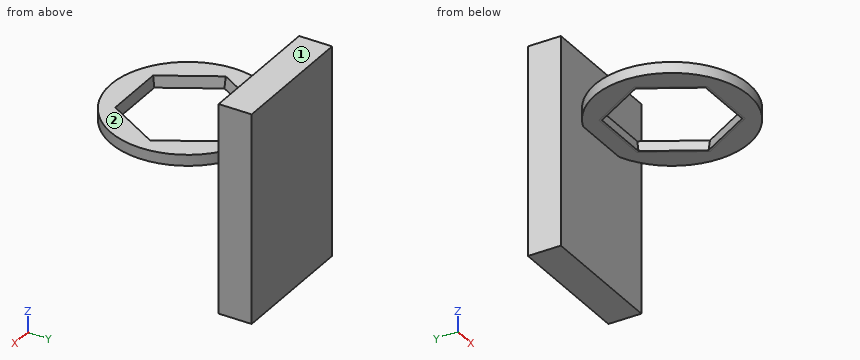
from build123d import *

# Parameters (mm, degrees)
ESQUISSE1_R               = 70
BOSS_EXTRU_1_DEPTH        = 10
CHANFREIN1_SIZE           = 10.000000024
CHANFREIN1_SIZE_2         = 1.74707794
D_PLACER_START            = -32.160153846
D_PLACER_LA_FACE1_DEPTH   = 61.565802755
D_PLACER_START_2          = -29.405648909
D_PLACER_LA_FACE1_2_DEPTH = 58.811297818
D_PLACER_LA_FACE1_3_DEPTH = 58.811297818
ESQUISSE2_W               = 120
ESQUISSE2_H               = 190
BOSS_EXTRU_2_DEPTH        = 30


with BuildPart() as part:
    # Esquisse1 → Boss.-Extru.1 (new body)
    with BuildSketch(Plane.XY):
        Circle(ESQUISSE1_R)
        Polygon((56.79394598, 0), (28.39697299, 49.185), (-28.39697299, 49.185), (-56.79394598, 0), (-28.39697299, -49.185), (28.39697299, -49.185), align=None, mode=Mode.SUBTRACT)
    extrude(amount=BOSS_EXTRU_1_DEPTH)

    # Chanfrein1
    # the kernel refuses this chamfer: 10.000000024, 1.74707794 mm, written as the material it takes off along each edge
    with BuildSketch(Plane(origin=(-54.38262227, -49.185, 10), x_dir=(0, 0, -1), z_dir=(1, 0, 0))) as chanfrein1_piece_1_section:
        Polygon((CHANFREIN1_SIZE, 0), (0, -CHANFREIN1_SIZE_2), (0, 0), align=None)
    chanfrein1_piece_1 = extrude(amount=108.76524454, mode=Mode.PRIVATE)
    chanfrein1_piece_1 = split(chanfrein1_piece_1, bisect_by=Plane(origin=(7.702074175, -85.029616205, 10), z_dir=(-0.8660254037844389, 0.4999999999999996, 0)), keep=Keep.TOP, mode=Mode.PRIVATE)
    chanfrein1_piece_1 = split(chanfrein1_piece_1, bisect_by=Plane(origin=(-34.89338531, -37.932883795, 10), z_dir=(0.8660254037844386, 0.5000000000000001, 0)), keep=Keep.TOP, mode=Mode.PRIVATE)
    add(chanfrein1_piece_1, mode=Mode.SUBTRACT)
    with BuildSketch(Plane(origin=(15.40414835, -71.68923241, 10), x_dir=(0, 0, -1), z_dir=(0.4999999999999996, 0.8660254037844389, 0))) as chanfrein1_piece_2_section:
        Polygon((CHANFREIN1_SIZE, 0), (0, -CHANFREIN1_SIZE_2), (0, 0), align=None)
    chanfrein1_piece_2 = extrude(amount=108.76524454, mode=Mode.PRIVATE)
    chanfrein1_piece_2 = split(chanfrein1_piece_2, bisect_by=Plane(origin=(15.40414835, -49.185, 10), z_dir=(0, 1, 0)), keep=Keep.TOP, mode=Mode.PRIVATE)
    chanfrein1_piece_2 = split(chanfrein1_piece_2, bisect_by=Plane(origin=(77.488844795, -35.844616205, 10), z_dir=(-0.8660254037844386, -0.5000000000000001, 0)), keep=Keep.TOP, mode=Mode.PRIVATE)
    add(chanfrein1_piece_2, mode=Mode.SUBTRACT)
    with BuildSketch(Plane(origin=(69.78677062, -22.50423241, 10), x_dir=(0, 0, -1), z_dir=(-0.5000000000000001, 0.8660254037844386, 0))) as chanfrein1_piece_3_section:
        Polygon((CHANFREIN1_SIZE, 0), (0, -CHANFREIN1_SIZE_2), (0, 0), align=None)
    chanfrein1_piece_3 = extrude(amount=108.76524454, mode=Mode.PRIVATE)
    chanfrein1_piece_3 = split(chanfrein1_piece_3, bisect_by=Plane(origin=(50.29753366, -11.252116205, 10), z_dir=(-0.8660254037844389, 0.4999999999999996, 0)), keep=Keep.TOP, mode=Mode.PRIVATE)
    chanfrein1_piece_3 = split(chanfrein1_piece_3, bisect_by=Plane(origin=(69.78677062, 49.185, 10), z_dir=(0, -1, 0)), keep=Keep.TOP, mode=Mode.PRIVATE)
    add(chanfrein1_piece_3, mode=Mode.SUBTRACT)
    with BuildSketch(Plane(origin=(54.38262227, 49.185, 10), x_dir=(0, 0, -1), z_dir=(-1, 0, 0))) as chanfrein1_piece_4_section:
        Polygon((CHANFREIN1_SIZE, 0), (0, -CHANFREIN1_SIZE_2), (0, 0), align=None)
    chanfrein1_piece_4 = extrude(amount=108.76524454, mode=Mode.PRIVATE)
    chanfrein1_piece_4 = split(chanfrein1_piece_4, bisect_by=Plane(origin=(-7.702074175, 85.029616205, 10), z_dir=(0.8660254037844388, -0.4999999999999998, 0)), keep=Keep.TOP, mode=Mode.PRIVATE)
    chanfrein1_piece_4 = split(chanfrein1_piece_4, bisect_by=Plane(origin=(34.89338531, 37.932883795, 10), z_dir=(-0.8660254037844386, -0.5000000000000001, 0)), keep=Keep.TOP, mode=Mode.PRIVATE)
    add(chanfrein1_piece_4, mode=Mode.SUBTRACT)
    with BuildSketch(Plane(origin=(-15.40414835, 71.68923241, 10), x_dir=(0, 0, -1), z_dir=(-0.4999999999999998, -0.8660254037844388, 0))) as chanfrein1_piece_5_section:
        Polygon((CHANFREIN1_SIZE, 0), (0, -CHANFREIN1_SIZE_2), (0, 0), align=None)
    chanfrein1_piece_5 = extrude(amount=108.76524454, mode=Mode.PRIVATE)
    chanfrein1_piece_5 = split(chanfrein1_piece_5, bisect_by=Plane(origin=(-77.488844795, 35.844616205, 10), z_dir=(0.8660254037844386, 0.5000000000000001, 0)), keep=Keep.TOP, mode=Mode.PRIVATE)
    chanfrein1_piece_5 = split(chanfrein1_piece_5, bisect_by=Plane(origin=(-15.40414835, 49.185, 10), z_dir=(0, -1, 0)), keep=Keep.TOP, mode=Mode.PRIVATE)
    add(chanfrein1_piece_5, mode=Mode.SUBTRACT)
    with BuildSketch(Plane(origin=(-69.78677062, 22.50423241, 10), x_dir=(0, 0, -1), z_dir=(0.5000000000000001, -0.8660254037844386, 0))) as chanfrein1_piece_6_section:
        Polygon((CHANFREIN1_SIZE, 0), (0, -CHANFREIN1_SIZE_2), (0, 0), align=None)
    chanfrein1_piece_6 = extrude(amount=108.76524454, mode=Mode.PRIVATE)
    chanfrein1_piece_6 = split(chanfrein1_piece_6, bisect_by=Plane(origin=(-69.78677062, -49.185, 10), z_dir=(0, 1, 0)), keep=Keep.TOP, mode=Mode.PRIVATE)
    chanfrein1_piece_6 = split(chanfrein1_piece_6, bisect_by=Plane(origin=(-50.29753366, 11.252116205, 10), z_dir=(0.8660254037844388, -0.4999999999999998, 0)), keep=Keep.TOP, mode=Mode.PRIVATE)
    add(chanfrein1_piece_6, mode=Mode.SUBTRACT)
    with BuildSketch(Plane(origin=(-54.38262227, -49.185, 10), x_dir=(0, 0, -1), z_dir=(1, 0, 0))) as chanfrein1_piece_7a_section:
        Polygon((CHANFREIN1_SIZE, 0), (0, -CHANFREIN1_SIZE_2), (0, 0), align=None)
    chanfrein1_piece_7a = extrude(amount=108.76524454, mode=Mode.PRIVATE)
    chanfrein1_piece_7a = split(chanfrein1_piece_7a, bisect_by=Plane(origin=(-34.89338531, -37.932883795, 10), z_dir=(-0.8660254037844386, -0.5000000000000001, 0)), keep=Keep.TOP, mode=Mode.PRIVATE)
    with BuildSketch(Plane(origin=(-69.78677062, 22.50423241, 10), x_dir=(0, 0, -1), z_dir=(0.5000000000000001, -0.8660254037844386, 0))) as chanfrein1_piece_7b_section:
        Polygon((CHANFREIN1_SIZE, 0), (0, -CHANFREIN1_SIZE_2), (0, 0), align=None)
    chanfrein1_piece_7b = extrude(amount=108.76524454, mode=Mode.PRIVATE)
    chanfrein1_piece_7b = split(chanfrein1_piece_7b, bisect_by=Plane(origin=(-69.78677062, -49.185, 10), z_dir=(0, -1, 0)), keep=Keep.TOP, mode=Mode.PRIVATE)
    chanfrein1_piece_7 = chanfrein1_piece_7a & chanfrein1_piece_7b
    add(chanfrein1_piece_7, mode=Mode.SUBTRACT)
    with BuildSketch(Plane(origin=(15.40414835, -71.68923241, 10), x_dir=(0, 0, -1), z_dir=(0.4999999999999996, 0.8660254037844389, 0))) as chanfrein1_piece_8a_section:
        Polygon((CHANFREIN1_SIZE, 0), (0, -CHANFREIN1_SIZE_2), (0, 0), align=None)
    chanfrein1_piece_8a = extrude(amount=108.76524454, mode=Mode.PRIVATE)
    chanfrein1_piece_8a = split(chanfrein1_piece_8a, bisect_by=Plane(origin=(15.40414835, -49.185, 10), z_dir=(0, -1, 0)), keep=Keep.TOP, mode=Mode.PRIVATE)
    with BuildSketch(Plane(origin=(-54.38262227, -49.185, 10), x_dir=(0, 0, -1), z_dir=(1, 0, 0))) as chanfrein1_piece_8b_section:
        Polygon((CHANFREIN1_SIZE, 0), (0, -CHANFREIN1_SIZE_2), (0, 0), align=None)
    chanfrein1_piece_8b = extrude(amount=108.76524454, mode=Mode.PRIVATE)
    chanfrein1_piece_8b = split(chanfrein1_piece_8b, bisect_by=Plane(origin=(7.702074175, -85.029616205, 10), z_dir=(0.8660254037844389, -0.4999999999999996, 0)), keep=Keep.TOP, mode=Mode.PRIVATE)
    chanfrein1_piece_8 = chanfrein1_piece_8a & chanfrein1_piece_8b
    add(chanfrein1_piece_8, mode=Mode.SUBTRACT)
    with BuildSketch(Plane(origin=(15.40414835, -71.68923241, 10), x_dir=(0, 0, -1), z_dir=(0.4999999999999996, 0.8660254037844389, 0))) as chanfrein1_piece_9a_section:
        Polygon((CHANFREIN1_SIZE, 0), (0, -CHANFREIN1_SIZE_2), (0, 0), align=None)
    chanfrein1_piece_9a = extrude(amount=108.76524454, mode=Mode.PRIVATE)
    chanfrein1_piece_9a = split(chanfrein1_piece_9a, bisect_by=Plane(origin=(77.488844795, -35.844616205, 10), z_dir=(0.8660254037844386, 0.5000000000000001, 0)), keep=Keep.TOP, mode=Mode.PRIVATE)
    with BuildSketch(Plane(origin=(69.78677062, -22.50423241, 10), x_dir=(0, 0, -1), z_dir=(-0.5000000000000001, 0.8660254037844386, 0))) as chanfrein1_piece_9b_section:
        Polygon((CHANFREIN1_SIZE, 0), (0, -CHANFREIN1_SIZE_2), (0, 0), align=None)
    chanfrein1_piece_9b = extrude(amount=108.76524454, mode=Mode.PRIVATE)
    chanfrein1_piece_9b = split(chanfrein1_piece_9b, bisect_by=Plane(origin=(50.29753366, -11.252116205, 10), z_dir=(0.8660254037844389, -0.4999999999999996, 0)), keep=Keep.TOP, mode=Mode.PRIVATE)
    chanfrein1_piece_9 = chanfrein1_piece_9a & chanfrein1_piece_9b
    add(chanfrein1_piece_9, mode=Mode.SUBTRACT)
    with BuildSketch(Plane(origin=(54.38262227, 49.185, 10), x_dir=(0, 0, -1), z_dir=(-1, 0, 0))) as chanfrein1_piece_10a_section:
        Polygon((CHANFREIN1_SIZE, 0), (0, -CHANFREIN1_SIZE_2), (0, 0), align=None)
    chanfrein1_piece_10a = extrude(amount=108.76524454, mode=Mode.PRIVATE)
    chanfrein1_piece_10a = split(chanfrein1_piece_10a, bisect_by=Plane(origin=(34.89338531, 37.932883795, 10), z_dir=(0.8660254037844386, 0.5000000000000001, 0)), keep=Keep.TOP, mode=Mode.PRIVATE)
    with BuildSketch(Plane(origin=(69.78677062, -22.50423241, 10), x_dir=(0, 0, -1), z_dir=(-0.5000000000000001, 0.8660254037844386, 0))) as chanfrein1_piece_10b_section:
        Polygon((CHANFREIN1_SIZE, 0), (0, -CHANFREIN1_SIZE_2), (0, 0), align=None)
    chanfrein1_piece_10b = extrude(amount=108.76524454, mode=Mode.PRIVATE)
    chanfrein1_piece_10b = split(chanfrein1_piece_10b, bisect_by=Plane(origin=(69.78677062, 49.185, 10), z_dir=(0, 1, 0)), keep=Keep.TOP, mode=Mode.PRIVATE)
    chanfrein1_piece_10 = chanfrein1_piece_10a & chanfrein1_piece_10b
    add(chanfrein1_piece_10, mode=Mode.SUBTRACT)
    with BuildSketch(Plane(origin=(-15.40414835, 71.68923241, 10), x_dir=(0, 0, -1), z_dir=(-0.4999999999999998, -0.8660254037844388, 0))) as chanfrein1_piece_11a_section:
        Polygon((CHANFREIN1_SIZE, 0), (0, -CHANFREIN1_SIZE_2), (0, 0), align=None)
    chanfrein1_piece_11a = extrude(amount=108.76524454, mode=Mode.PRIVATE)
    chanfrein1_piece_11a = split(chanfrein1_piece_11a, bisect_by=Plane(origin=(-15.40414835, 49.185, 10), z_dir=(0, 1, 0)), keep=Keep.TOP, mode=Mode.PRIVATE)
    with BuildSketch(Plane(origin=(54.38262227, 49.185, 10), x_dir=(0, 0, -1), z_dir=(-1, 0, 0))) as chanfrein1_piece_11b_section:
        Polygon((CHANFREIN1_SIZE, 0), (0, -CHANFREIN1_SIZE_2), (0, 0), align=None)
    chanfrein1_piece_11b = extrude(amount=108.76524454, mode=Mode.PRIVATE)
    chanfrein1_piece_11b = split(chanfrein1_piece_11b, bisect_by=Plane(origin=(-7.702074175, 85.029616205, 10), z_dir=(-0.8660254037844388, 0.4999999999999998, 0)), keep=Keep.TOP, mode=Mode.PRIVATE)
    chanfrein1_piece_11 = chanfrein1_piece_11a & chanfrein1_piece_11b
    add(chanfrein1_piece_11, mode=Mode.SUBTRACT)
    with BuildSketch(Plane(origin=(-69.78677062, 22.50423241, 10), x_dir=(0, 0, -1), z_dir=(0.5000000000000001, -0.8660254037844386, 0))) as chanfrein1_piece_12a_section:
        Polygon((CHANFREIN1_SIZE, 0), (0, -CHANFREIN1_SIZE_2), (0, 0), align=None)
    chanfrein1_piece_12a = extrude(amount=108.76524454, mode=Mode.PRIVATE)
    chanfrein1_piece_12a = split(chanfrein1_piece_12a, bisect_by=Plane(origin=(-50.29753366, 11.252116205, 10), z_dir=(-0.8660254037844388, 0.4999999999999998, 0)), keep=Keep.TOP, mode=Mode.PRIVATE)
    with BuildSketch(Plane(origin=(-15.40414835, 71.68923241, 10), x_dir=(0, 0, -1), z_dir=(-0.4999999999999998, -0.8660254037844388, 0))) as chanfrein1_piece_12b_section:
        Polygon((CHANFREIN1_SIZE, 0), (0, -CHANFREIN1_SIZE_2), (0, 0), align=None)
    chanfrein1_piece_12b = extrude(amount=108.76524454, mode=Mode.PRIVATE)
    chanfrein1_piece_12b = split(chanfrein1_piece_12b, bisect_by=Plane(origin=(-77.488844795, 35.844616205, 10), z_dir=(-0.8660254037844386, -0.5000000000000001, 0)), keep=Keep.TOP, mode=Mode.PRIVATE)
    chanfrein1_piece_12 = chanfrein1_piece_12a & chanfrein1_piece_12b
    add(chanfrein1_piece_12, mode=Mode.SUBTRACT)

    # Déplacer la face1: read off the stored shape, not the designer's step
    # Déplacer la face1 outline → Déplacer la face1 (add)
    with BuildSketch(Plane.YZ.offset(D_PLACER_START)):
        Polygon((49.185000004, -1e-09), (50.93207794, 10), (48.901784549, 10), (47.154706614, 0), align=None)
        Polygon((-47.154706614, 0), (-48.901784549, 10), (-50.93207794, 10), (-49.185000004, -1e-09), align=None)
    extrude(amount=D_PLACER_LA_FACE1_DEPTH)

    # D_placer la face1 2 outline → D_placer la face1 2 (add)
    with BuildSketch(Plane(origin=(0, 0, 0), x_dir=(0.8660254037844389, -0.49999999999999956, 0), z_dir=(0.4999999999999996, 0.8660254037844388, 0)).offset(D_PLACER_START_2)):
        Polygon((-49.185000004, 1e-09), (-50.93207794, -10), (-48.901784549, -10), (-47.154706614, 0), align=None)
        Polygon((47.154706614, 0), (48.901784549, -10), (50.93207794, -10), (49.185000004, 1e-09), align=None)
    extrude(amount=D_PLACER_LA_FACE1_2_DEPTH)

    # D_placer la face1 3 outline → D_placer la face1 3 (add)
    with BuildSketch(Plane(origin=(0, 0, 0), x_dir=(0.8660254037844386, 0.5000000000000001, 0), z_dir=(0.5000000000000001, -0.8660254037844386, 0)).offset(D_PLACER_START_2)):
        Polygon((49.185000004, -1e-09), (50.93207794, 10), (48.901784549, 10), (47.154706614, 0), align=None)
        Polygon((-47.154706614, 0), (-48.901784549, 10), (-50.93207794, 10), (-49.185000004, -1e-09), align=None)
    extrude(amount=D_PLACER_LA_FACE1_3_DEPTH)

    # Esquisse2 → Boss.-Extru.2 (add)
    with BuildSketch(Plane(origin=(0, 94.56764827, 0), x_dir=(1, 0, 0), z_dir=(0, 1, 0))):
        with Locations((0, 30)):
            Rectangle(ESQUISSE2_W, ESQUISSE2_H)
    extrude(amount=-BOSS_EXTRU_2_DEPTH)


solid = part.part
The model under review builds one solid part; all positions refer to its coordinate system, in mm. Face numbers are marked on the shaded views. A direction names the side the tool comes from. Round coordinates to 2 decimals unless told otherwise and drop trailing zeros. Loops run counter-clockwise (first coordinate to the right, second up) from the corner with the lowest first, then second, coordinate; pieces in that order, holes last. Notation, with made-up numbers: (-15.75, 48) -> (9.25, 48) arc R23 cw to (9.25, 71) -> close; hole circle Ø4 at (25.25, 42). An arc over 180 degrees is marked (long way). One line per question, with ' | ' between items. Start each with the question number.
Item 1: Machinability: for the marked faces 1 and 2, which of the approach directions +Z, -Z, +X, -X, +Y, -Y give a long, thin tool a straight path to every point of the face, cutting with its end or side? Answer none if there is none.
Item 2: Add section D-D, the plane y = 32.5. Write out the cut boundary in (x, z), then the cut area to 3 significant figures.
Item 3: Add section C-C, the plane x = 34. Write out the cut boundary in (y, z), then the cut area to 3 significant figures.
Item 4: Wall thickness on line 1 along Y through (x, z) = (26, -3); line 2 along Y through (x, z) = (1.5, 8.5); line 3 along Z through (x, y) = (61, 27): over which ranges is each line inside the solid? List them lowest first. Write a range as [from, to].
Item 5: Add section B-B, the plane y = -9. Write out the cut boundary in (x, z), then the cut area to 3 significant figures.
Item 6: Add section A-A, the plane x = 0. Write out the cut boundary in (y, z) (3 decimals).
Item 7: For pin 1 (1 mm diameter, centred on x = 35.5, z = 28, fed in from -Y); pin 2 (2 mm diameter, centred on x = -11, y = -48.5, fed in from -Z); pin 3 (15 mm diameter, centred on y = 76, z = 17.5, fed in from +X), all flat-tipped, find the tip position at first contact; note any pin that passes through.
Return value:
1) face 1: +Z, +X, -X, +Y, -Y | face 2: +Z, +X, -X, -Y
2) outline: (-62, 0) -> (-35.69, 0) -> (-37.7, 10) -> (-62, 10) -> close; (35.69, 0) -> (62, 0) -> (62, 10) -> (37.7, 10) -> close | area: 506 mm2
3) outline: (-61.19, 0) -> (-35.42, 0) -> (-38.91, 10) -> (-61.19, 10) -> close; (35.42, 0) -> (61.19, 0) -> (61.19, 10) -> (38.91, 10) -> close; (64.57, -125) -> (94.57, -125) -> (94.57, 65) -> (64.57, 65) -> close | area: 6,180 mm2
4) line 1: y = [64.57, 94.57] | line 2: y = [-69.98, -48.64], [48.64, 94.57] | line 3: z = [0, 10]
5) outline: (-69.42, 0) -> (-49.25, 0) -> (-51.27, 10) -> (-69.42, 10) -> close; (49.25, 0) -> (69.42, 0) -> (69.42, 10) -> (51.27, 10) -> close | area: 383 mm2
6) outline: (-70, 0) -> (-47.155, 0) -> (-48.902, 10) -> (-70, 10) -> close; (47.155, 0) -> (64.568, 0) -> (64.568, -125) -> (94.568, -125) -> (94.568, 65) -> (64.568, 65) -> (64.568, 10) -> (48.902, 10) -> close
7) pin 1: stops at y = 64.57 | pin 2: stops at z = 0 | pin 3: stops at x = 60
